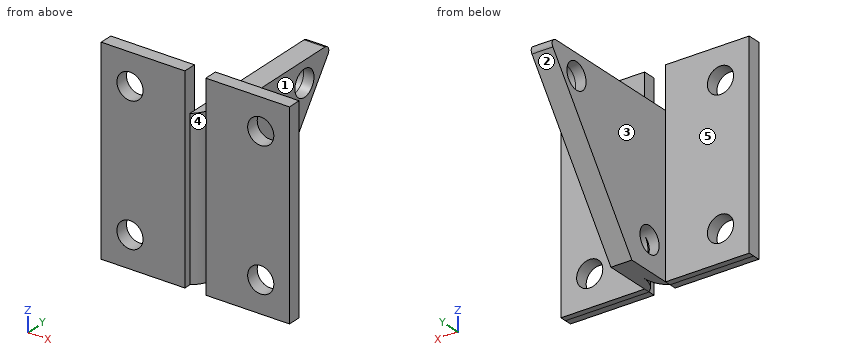
from build123d import *

# Parameters (mm, degrees)
SKETCH1_R            = 2.5
BOSS_EXTRUDE2_DEPTH  = 2
BOSS_EXTRUDE4_DEPTH  = 16
FILLET1_R            = 5
FILLET1_OF_MIRROR1_R = 5
SKETCH3_R            = 2.5
CUT_EXTRUDE2_DEPTH   = 78.57995838
FILLET2_R            = 1


with BuildPart() as part:
    # Sketch1 → Boss-Extrude2 (new body)
    with BuildSketch(Plane(origin=(0, 0, 0), x_dir=(0, 0, -1), z_dir=(1, 0, 0))):
        Polygon((-60.951444932, 12.55580533), (-30.968352486, -9.282744271), (-30.951444932, -19.282744271), (-60.951444932, -19.282744271), align=None)
        with Locations(Location((-36.501270434, -13.912745065, 0), (0, 0, 180))):
            Circle(SKETCH1_R, mode=Mode.SUBTRACT)
        with Locations(Location((-56.951444932, 5.21290167, 0), (0, 0, 180))):
            Circle(SKETCH1_R, mode=Mode.SUBTRACT)
    boss_extrude2 = extrude(amount=BOSS_EXTRUDE2_DEPTH)

    # Sketch2 → Boss-Extrude4 (add)
    with BuildSketch(Plane(origin=(2, 0, 0), x_dir=(0, 0, -1), z_dir=(1, 0, 0))):
        Polygon((-68.951444932, -20.609291835), (-68.951444932, -19.609291835), (-68.951444932, -18.109291835), (-30.953428953, -18.109291835), (-30.951444932, -19.282744271), (-30.951444932, -20.609291835), align=None)
    boss_extrude4 = extrude(amount=BOSS_EXTRUDE4_DEPTH)

    # Fillet1
    # the kernel refuses this fillet: 5 mm, written as the material it takes off along each edge
    with BuildSketch(Plane(origin=(0, -19.282744271, 20.951444932), x_dir=(0, 1, 0), z_dir=(0, 0, 1))) as fillet1_piece_1:
        with BuildLine():
            CenterArc((4, -5), FILLET1_R, 90, 53.130102354)
            Line((0, -2), (-0.08, -1.94))
            ThreePointArc((-0.08, -1.94), (-0.1, -1), (-0.1, 0))
            Line((-0.1, 0), (0, 0.1))
            Line((0, 0.1), (4, 0.1))
            Line((4, 0.1), (4, 0))
        make_face()
    extrude(amount=50, mode=Mode.SUBTRACT)


with BuildPart() as mirror1_1:
    # Mirror1: Boss-Extrude2, Boss-Extrude4 across plane
    add(boss_extrude2.mirror(Plane(origin=(0, 0, 0), x_dir=(0, 0, 1), z_dir=(1, 0, 0))))
    add(boss_extrude4.mirror(Plane(origin=(0, 0, 0), x_dir=(0, 0, 1), z_dir=(1, 0, 0))))

    # Fillet1 of Mirror1
    # the kernel refuses this fillet: 5 mm, written as the material it takes off along each edge
    with BuildSketch(Plane(origin=(0, -19.282744271, 20.951444932), x_dir=(0, 1, 0), z_dir=(0, 0, 1))) as fillet1_of_mirror1_piece_1:
        with BuildLine():
            CenterArc((4, 5), FILLET1_OF_MIRROR1_R, 216.869897646, 53.130102354)
            Line((0, 2), (-0.08, 1.94))
            ThreePointArc((-0.08, 1.94), (-0.1, 1), (-0.1, 0))
            Line((-0.1, 0), (0, -0.1))
            Line((0, -0.1), (4, -0.1))
            Line((4, -0.1), (4, 0))
        make_face()
    extrude(amount=50, mode=Mode.SUBTRACT)


with BuildPart() as part_1:
    add(part.part)

    # Mirror1 united with what the copies touc: union Mirror1_1
    add(mirror1_1.part)

    # Sketch3 → Cut-Extrude2 (cut, through all)
    with BuildSketch(Plane(origin=(0, -18.109291835, 0), x_dir=(1, 0, 0), z_dir=(0, 1, 0))):
        with Locations(Location((12.5, -62.953428953, 0), (0, 0, 270))):
            Circle(SKETCH3_R)
        with Locations(Location((12.5, -36.953428953, 0), (0, 0, 270))):
            Circle(SKETCH3_R)
    cut_extrude2 = extrude(amount=-CUT_EXTRUDE2_DEPTH, mode=Mode.SUBTRACT)

    # Mirror2: Cut-Extrude2 across plane
    add(cut_extrude2.mirror(Plane(origin=(0, 0, 0), x_dir=(0, 0, 1), z_dir=(1, 0, 0))), mode=Mode.SUBTRACT)

    # Fillet2
    fillet2_edges = [part_1.edges().sort_by_distance(p)[0] for p in [
        (0, 12.55580533, 60.951444932),
    ]]
    fillet(fillet2_edges, radius=FILLET2_R)


solid = part_1.part
Design review of the part built by this model. Coordinates are the model's own, in mm. Face numbers are marked on the shaded views. A direction names the side the tool comes from. Round coordinates to 2 decimals unless told otherwise and drop trailing zeros. Write each loop counter-clockwise with the first axis right and the second up, starting at its lowest first coordinate (ties: lowest second). Pieces come first, ordered by that corner, then holes. Notation, with made-up numbers: M -36,32 L 17,32 A7 ccw 17,41 Z; hole C 72.25,9.25 d3. An arc over 180 degrees is marked long. One line per item, written item: value. Start each with the question number.
1. Take a section at A-A on z = 64. State the section outline as (x, y) points, then the cut area to 3 significant figures.
2. Draft analysis for pull direction X (two halves, no side actions). For the marked faces 3, 4 and 5, state which applies: pulls with the +X half, pulls with the -X half, needs draft (parallel to the pull), parting line crosses it, or undercut.
3. Take a section at C-C on z = 45.5. State the section outline as (x, y) points, then the cut area to 3 significant figures.
4. To check wall thickness, follow probe 1 along Z at (x, y) = (-12.5, -19.85); probe 2 along Z at (x, y) = (-12, -19); probe 3 along X at (y, z) = (3, 59). State the ranges of each line that lie inside material, in increasing order. Write a range as from..to.
5. Take a section at D-D on x = -16. State the section outline as (y, z) points.
6. Take a section at B-B on x = 12.5. State the section outline as (y, z) points, then the cut area to 3 significant figures.
7. For the marked faces 1 and 2, list the 3-axis set-ups (+Z, -Z, +X, -X, +Y, -Y) from which the entire face can be reached by the end or side of a thin tool; tool diameter is ignored.
8. Clearance check with flat-ended pins moving along their axes: P1, Ø4.5, axis at x = -0.5, y = -10.5, coming from the +Z side; P2, Ø8, axis at y = 5.21, z = 56.95, coming from the +X side; P3, Ø6, axis at y = -13.91, z = 36.5, coming from the -X side. State where each tip first meets the part, or that it passes through.
Computed:
1. outline: M -18,-20.61 L -14.77,-20.61 L -14.77,-18.11 L -18,-18.11 Z; M -10.23,-20.61 L -2,-20.61 L -2,-18.11 L -10.23,-18.11 Z; M 2,-20.61 L 10.23,-20.61 L 10.23,-18.11 L 2,-18.11 Z; M 14.77,-20.61 L 18,-20.61 L 18,-18.11 L 14.77,-18.11 Z
1. area: 57.3 mm²
2. face 3: pulls with the -X half
2. face 4: undercut
2. face 5: needs draft
3. outline: M -18,-20.61 L -2,-20.61 L -2,-19.28 A5 ccw 0,-15.28 A5 ccw 2,-19.28 L 2,-20.61 L 18,-20.61 L 18,-18.11 L 2,-18.11 L 2,1.3 L -2,1.3 L -2,-18.11 L -18,-18.11 Z
3. area: 158 mm²
4. probe 1: z = 30.95..34.45, 39.45..60.45, 65.45..68.95
4. probe 2: z = 30.95..34.5, 39.4..60.5, 65.4..68.95
4. probe 3: x = -2..2
5. outline: M -20.61,30.95 L -19.28,30.95 L -18.11,30.95 L -18.11,68.95 L -20.61,68.95 Z
6. outline: M -20.61,30.95 L -19.28,30.95 L -18.11,30.95 L -18.11,34.45 L -20.61,34.45 Z; M -20.61,39.45 L -18.11,39.45 L -18.11,60.45 L -20.61,60.45 Z; M -20.61,65.45 L -18.11,65.45 L -18.11,68.95 L -20.61,68.95 Z
6. area: 70.0 mm²
7. face 1: +Z, -Z, +X, +Y
7. face 2: -Z, +X, -X, +Y
8. P1: stops at z = 60.95
8. P2: stops at x = 2
8. P3: stops at x = -2
